Input: part model. Units: mm. Frame: model coordinates. A direction names the side the tool comes from. Round coordinates to 2 decimals unless told otherwise and drop trailing zeros. Loops run counter-clockwise (first coordinate to the right, second up) from the corner with the lowest first, then second, coordinate; pieces in that order, holes last. Notation, with made-up numbers: (-34.75, 75) -> (-3.75, 75) arc R19 ccw to (-3.75, 85) -> close; hole circle Ø3 at (21.25, 17). An arc over 180 degrees is marked (long way). Answer as a JSON object with one key per item and string values. Group by question number.
Item 1: Pin query (flat end, axial travel): pin 1 (0.6 mm diameter, centred on y = -6.5, z = 17.5, fed in from -X); pin 2 (0.6 mm diameter, centred on x = 39.5, y = 6, fed in from +Z); pin 3 (0.6 mm diameter, centred on y = -6.5, z = 17, fed in from +X). Return the tip coordinate at first contact, or that it passes through.
Item 2: Material intervals for line 1 (X direction, y = -4.25, z = 15); line 2 (Y direction, x = -10, z = 3); line 3 (Z direction, x = -3, y = -0.25), sorted ascending. Write a range as [from, to].
Item 3: Section query B-B on z = 4.5. Return loops of the section in (x, y).
Item 4: Section query A-A on x = 40. Return loops of the section in (y, z).
Item 5: Draft query along Y for faces 3 (the cylindrical face through (-45.232, 0.063, 23.574)), 4 (the cylindrical face through (-44.9, 0.1, 23.2)), 5 (the cylindrical face through (-46.17, 5.87, 10.14)), 6 (the cylindrical face through (46.13, -5.91, 9.86)). Return one class per face: released by +Y, released by -Y, zero draft, split by the parting line, or undercut.
Item 6: Section query D-D on x = -32. Return loops of the section in (y, z), and give its area (3 significant figures).
Item 7: Set-up query: faces 1 (the cylindrical face through (0.584, 5.874, 24.43)), 2 (the flat face through (-46.236, 0, 10)). Return all of +Z, -Z, +X, -X, +Y, -Y with unobstructed straight access to the full face (end or side cutting, diameter ignored); none if empty.
Item 8: Section query C-C on y = 0.5. Return loops of the section in (x, z), and give its area (3 significant figures).
from build123d import *

# Parameters (mm, degrees)
F0_W     = 93.4718027711
F0_H     = 12.9508469254
F1_DEPTH = 25
F2_R     = 5
F3_R     = 5
F4_R     = 2
F5_T     = -0.5
F6_W     = 5.4559892522
F6_H     = 6.0577589622
F6_W_2   = 4.9121007323
F6_H_2   = 5.9622740373
F6_W_3   = 6.1655344907
F6_H_3   = 5.8267693967
F7_DEPTH = 10
F8_W     = 9.2564252019
F8_H     = 7.081441097
F9_DEPTH = 5


with BuildPart() as f1:
    # F0 (on Top) → F1 (new body)
    with BuildSketch(Plane.XY):
        Rectangle(F0_W, F0_H)
    extrude(amount=F1_DEPTH)

    # F2
    f2_edges = [f1.edges().sort_by_distance(p)[0] for p in [
        (46.735901, 0, 25),
    ]]
    fillet(f2_edges, radius=F2_R)

    # F3
    f3_edges = [f1.edges().sort_by_distance(p)[0] for p in [
        (-46.735901, 0, 25),
    ]]
    fillet(f3_edges, radius=F3_R)

    # F4
    f4_edges = [f1.edges().sort_by_distance(p)[0] for p in [
        (0, -6.475423, 25),
        (0, 6.475423, 25),
        (46.735901, 6.475423, 10),
        (46.735901, -6.475423, 10),
        (-46.735901, -6.475423, 10),
        (-45.271435, -6.475423, 23.535534),
        (45.271435, -6.475423, 23.535534),
        (-45.271435, 6.475423, 23.535534),
        (45.271435, 6.475423, 23.535534),
        (-46.735901, 6.475423, 10),
    ]]
    fillet(f4_edges, radius=F4_R)

    # F5
    f5_openings = [f1.faces().sort_by_distance(p)[0] for p in [
        (0, 0, 0),
    ]]
    offset(amount=F5_T, openings=f5_openings)

    # F6 (on face) → F7 (cut)
    with BuildSketch(Plane.XZ.offset(6.4754234627)):
        with Locations((-39.0079067595, 16.9711205189)):
            Rectangle(F6_W, F6_H)
        with Locations((-30.8063998818, 17.0389381237)):
            Rectangle(F6_W_2, F6_H_2)
        Polygon((-25.5047174612, 20.0200751424), (-25.5047174612, 14.1596693691), (-20.3863596622, 14.2051883272), (-20.43789451, 20), align=None)
        Polygon((-16.4258014411, 20.155582577), (-16.3241717964, 14.3288131803), (-10.9716746956, 14.3288131803), (-10.9716746956, 20.155582577), align=None)
        with Locations((-4.5351273147, 17.2421978787)):
            Rectangle(F6_W_3, F6_H_3)
        Polygon((2.711430509, 20.2894311491), (2.711430509, 14.4981949606), (8.747510295, 14.4981949606), (8.747510295, 20.4250746066), align=None)
        Polygon((19.1331994785, 20.2894311491), (13.6082590709, 20.2894311491), (13.6082590709, 14.5744122565), (19.308578223, 14.5405353978), align=None)
        Polygon((22.3996791117, 20.4367674267), (22.5268509239, 14.7776724771), (27.8793480247, 14.7776724771), (27.7521591139, 20.4375283061), align=None)
        Polygon((30.7136761403, 20.5000031751), (30.8842776962, 14.9077031341), (35.1938740726, 15.0391738782), (35.0232725167, 20.6314739191), align=None)
    extrude(amount=-F7_DEPTH, mode=Mode.SUBTRACT)

    # F8 (on face) → F9 (cut)
    with BuildSketch(Plane(origin=(0, 6.4754234627, 0), x_dir=(-1, 0, 0), z_dir=(0, 1, 0))):
        with Locations((-37.1076887846, 16.4592794515)):
            Rectangle(F8_W, F8_H)
        with Locations((-20.3512632847, 13.3706254326)):
            Rectangle(F8_W, F8_H)
    extrude(amount=-F9_DEPTH, mode=Mode.SUBTRACT)


solid = f1.part
Solved:
{
 "1": {"pin 1": "x = -45.75", "pin 2": "z = 24.58", "pin 3": "x = 45.75"},
 "2": {"line 1": "[-46.74, -46.24], [46.24, 46.74]", "line 2": "[-6.48, -5.98], [5.98, 6.48]", "line 3": "[24.5, 25]"},
 "3": {"outline": "(-46.74, -4.48) arc R2 ccw to (-44.74, -6.48) -> (44.74, -6.48) arc R2 ccw to (46.74, -4.48) -> (46.74, 4.48) arc R2 ccw to (44.74, 6.48) -> (-44.74, 6.48) arc R2 ccw to (-46.74, 4.48) -> close; hole (-46.24, -4.48) arc R1.5 ccw to (-44.74, -5.98) -> (44.74, -5.98) arc R1.5 ccw to (46.24, -4.48) -> (46.24, 4.48) arc R1.5 ccw to (44.74, 5.98) -> (-44.74, 5.98) arc R1.5 ccw to (-46.24, 4.48) -> close"},
 "4": {"outline": "(-6.48, 0) -> (-5.98, 0) -> (-5.98, 23) arc R1.5 cw to (-4.48, 24.5) -> (4.48, 24.5) arc R1.5 cw to (5.98, 23) -> (5.98, 20) -> (6.48, 20) -> (6.48, 23) arc R2 ccw to (4.48, 25) -> (-4.48, 25) arc R2 ccw to (-6.48, 23) -> close; (5.98, 0) -> (6.48, 0) -> (6.48, 12.92) -> (5.98, 12.92) -> close"},
 "5": {"face 3": "zero draft", "face 4": "undercut", "face 5": "released by +Y", "face 6": "released by -Y"},
 "6": {"outline": "(-6.48, 0) -> (-5.98, 0) -> (-5.98, 14.06) -> (-6.48, 14.06) -> close; (-6.48, 20.02) -> (-5.98, 20.02) -> (-5.98, 23) arc R1.5 cw to (-4.48, 24.5) -> (4.48, 24.5) arc R1.5 cw to (5.98, 23) -> (5.98, 0) -> (6.48, 0) -> (6.48, 23) arc R2 ccw to (4.48, 25) -> (-4.48, 25) arc R2 ccw to (-6.48, 23) -> close", "area": "27.2 mm²"},
 "7": {"face 1": "+Z, +X, -X, +Y", "face 2": "-Z"},
 "8": {"outline": "(-46.74, 0) -> (-46.24, 0) -> (-46.24, 20) arc R4.5 cw to (-41.74, 24.5) -> (41.74, 24.5) arc R4.5 cw to (46.24, 20) -> (46.24, 0) -> (46.74, 0) -> (46.74, 20) arc R5 ccw to (41.74, 25) -> (-41.74, 25) arc R5 ccw to (-46.74, 20) -> close", "area": "69.2 mm²"}
}
